from build123d import *

# Parameters (mm, degrees)
SKETCH1_W           = 127
SKETCH1_H           = 12.7
SKETCH1_R           = 4.7625
SKETCH1_R_2         = 2.38125
BOSS_EXTRUDE1_DEPTH = 3.175
SKETCH2_R           = 1.1303
CUT_EXTRUDE1_DEPTH  = 6.35


with BuildPart() as part:
    # Sketch1 → Boss-Extrude1 (new body)
    with BuildSketch(Plane.XY):
        with Locations((63.5, 6.35)):
            Rectangle(SKETCH1_W, SKETCH1_H)
        with Locations((6.35, 6.35)):
            Circle(SKETCH1_R, mode=Mode.SUBTRACT)
        with Locations((120.65, 6.35)):
            Circle(SKETCH1_R_2, mode=Mode.SUBTRACT)
    extrude(amount=BOSS_EXTRUDE1_DEPTH)

    # Sketch2 → Cut-Extrude1 (cut)
    with BuildSketch(Plane(origin=(0, 12.7, 0), x_dir=(1, 0, 0), z_dir=(0, 1, 0))):
        with Locations(Location((6.35, -1.5875, 0), (0, 0, 270))):
            Circle(SKETCH2_R)
    extrude(amount=-CUT_EXTRUDE1_DEPTH, mode=Mode.SUBTRACT)


solid = part.part
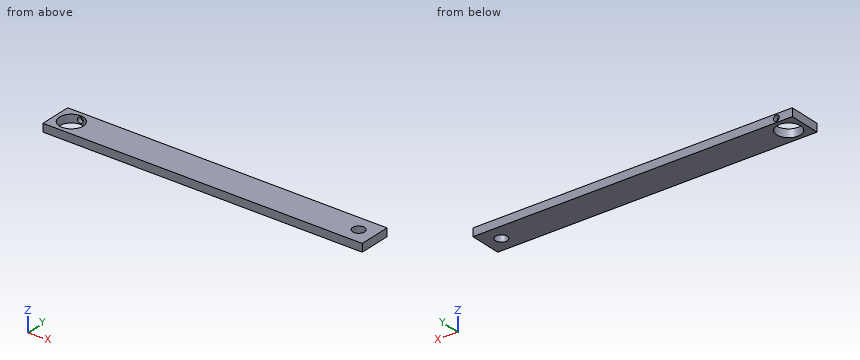
Model file for the job. Use its own axes, mm. Round coordinates to 2 decimals unless told otherwise and drop trailing zeros. Order: outer loops, then holes, each group sorted by start corner. A loop starts at its lowest first (then second) coordinate and runs counter-clockwise, first axis right, second up.
(1) Band-saw the part on A-A (x = 120.65). List the corners of the cut face in (y, z) (3 decimals).
(2) Band-saw the part on C-C (x = 6.35). List the corners of the cut face in (y, z) (1 decimal).
(3) Drill centre lines: line 1 (Z direction, x = 6.35, y = 11.5) (3 decimals); line 2 (Y direction, x = 120.65, z = 1.4); line 3 (X direction, y = 8.5, z = 2.95). Where is each one in solid material? Low to high.
(4) Band-saw the part on B-B (y = 6.35). List the corners of the cut face in (x, z) (1 decimal).
Verdict:
1. outline: (0, 0) - (3.969, 0) - (3.969, 3.175) - (0, 3.175) - close; (8.731, 0) - (12.7, 0) - (12.7, 3.175) - (8.731, 3.175) - close
2. outline: (0, 0) - (1.6, 0) - (1.6, 3.2) - (0, 3.2) - close; (11.1, 0) - (12.7, 0) - (12.7, 0.5) - (11.1, 0.5) - close; (11.1, 2.7) - (12.7, 2.7) - (12.7, 3.2) - (11.1, 3.2) - close
3. line 1: z = 0 to 0.457, 2.718 to 3.175
3. line 2: y = 0 to 3.97, 8.73 to 12.7
3. line 3: x = 0 to 2.1, 10.6 to 119.63, 121.67 to 127
4. outline: (0, 0) - (1.6, 0) - (1.6, 3.2) - (0, 3.2) - close; (11.1, 0) - (118.3, 0) - (118.3, 3.2) - (11.1, 3.2) - close; (123, 0) - (127, 0) - (127, 3.2) - (123, 3.2) - close
